Autodesk Inventor part; units mm, degrees
ref_plane "YZ Plane" through (0, 0, 0) normal (1, 0, 0) x (0, 1, 0)
ref_plane "XZ Plane" through (0, 0, 0) normal (0, 1, 0) x (-1, 0, 0)
ref_plane "XY Plane" through (0, 0, 0) normal (0, 0, 1) x (1, 0, 0)
sketch "Sketch6" plane through (0, 0, 0) normal (0, 0, 1) x (1, 0, 0)
  line L0 (40.1, 14.2) -> (56.7, 14.2)
  line L1 (56.7, 14.2) -> (56.7, -14.2)
  line L2 (56.7, -14.2) -> (40.1, -14.2)
  line L3 (40.1, -14.2) -> (40.1, 14.2)
  line L4 (35.6, -18.7) -> (61.2, -18.7)
  line L5 (61.2, -18.7) -> (61.2, 18.7)
  line L6 (61.2, 18.7) -> (35.6, 18.7)
  line L7 (35.6, 18.7) -> (35.6, -18.7)
  line L8 (-40.1, 14.2) -> (-56.7, 14.2)
  line L9 (-56.7, 14.2) -> (-56.7, -14.2)
  line L10 (-56.7, -14.2) -> (-40.1, -14.2)
  line L11 (-40.1, -14.2) -> (-40.1, 14.2)
  line L12 (-35.6, -18.7) -> (-61.2, -18.7)
  line L13 (-61.2, -18.7) -> (-61.2, 18.7)
  line L14 (-61.2, 18.7) -> (-35.6, 18.7)
  line L15 (-35.6, 18.7) -> (-35.6, -18.7)
  point P0 (35.6, 0)
  point P1 (35.6, 0)
  point P2 (-35.6, 0)
  point P3 (-35.6, 0)
extrude "Extrusion4" add sketch "Sketch6" along normal blind 40
sketch "Sketch7" plane through (0, 0, 0) normal (0, 0, -1) x (-1, 0, 0)
  line L0 (-35.6, -18.7) -> (-61.2, -18.7) construction
  line L1 (61.2, 18.7) -> (-61.2, 18.7)
  line L2 (-61.2, 18.7) -> (-61.2, -18.7)
  line L3 (-61.2, -18.7) -> (61.2, -18.7)
  line L4 (61.2, -18.7) -> (61.2, 18.7)
  point P0 (0, 0)
extrude "Extrusion5" add sketch "Sketch7" along normal blind 4.5
sketch "Sketch8" plane through (35.6, 18.7, 40) normal (0, 1, 0) x (1, 0, 0)
  line L0 (-71.2, 40) -> (0, 40) construction
  line L1 (0, 40) -> (0, 0) construction
  line L2 (-25.6, 40) -> (0, 0)
  line L3 (0, 11.1306) -> (-18.4764, 40)
  line L4 (-25.6, 40) -> (-18.4764, 40)
  line L5 (0, 11.1306) -> (0, 0)
  point P0 (-35.6, 40)
extrude "Extrusion6" add sketch "Sketch8" against normal blind 4.5
mirror "Mirror3" about plane through (0, 0, 0) normal (0, 1, 0) of "Extrusion6"
mirror "Mirror4" about plane through (0, 0, 0) normal (1, 0, 0) of "Extrusion6", "Mirror3"
sketch "Sketch9" plane through (0, 0, 0) normal (0, 0, 1) x (1, 0, 0)
  line L0 (12, -18.7) -> (12, -6.7)
  line L1 (-12, -6.7) -> (-12, -18.7)
  line L2 (-35.6, -18.7) -> (-10, -18.7) construction
  line L3 (12, -6.7) -> (-12, -6.7)
  line L4 (12, -18.7) -> (-12, -18.7)
  point P0 (0, 0)
extrude "Extrusion7" cut sketch "Sketch9" along normal mid plane 10
sketch "Sketch10" plane through (0, 0, -4.5) normal (0, 0, -1) x (-1, 0, 0)
  line L0 (12, -6.7) -> (-12, -6.7) construction
  line L1 (10, 18.7) -> (-10, 18.7) construction
  circle A0 centre (0, 12.35) radius 1.8
  circle A1 centre (0, -0.35) radius 1.8
  point P0 (0, 0)
extrude "Extrusion8" cut sketch "Sketch10" against normal blind 10
properties part number "Tablet_joint_Holder"
Model file for the job. Use its own axes, mm. A direction names the side the tool comes from. Coordinates: 2 decimals unless noted, no trailing zeros. Loops run counter-clockwise (first coordinate to the right, second up) from the corner with the lowest first, then second, coordinate; pieces in that order, holes last. Notation, with made-up numbers: (37, -0.5) - (50, -0.5) arc R24 ccw to (50, 31.5) - close; hole circle Ø7 at (70, -30.5). An arc over 180 degrees is marked (long way). Write item = value, one per line. Start each with the question number.
Item 1: Wall check: probe 1 along X at (y, z) = (2.5, 17); probe 2 along Y at (x, z) = (0, -2.5); probe 3 along Y at (x, z) = (31, 23). Give the ranges that are in metal, low to high. Write a range as [from, to].
Item 2: Saw through at B-B, the plane y = -8.5. List the corners of the cut face in (x, z).
Item 3: Drop flat-ended pins along their axis: pin 1 Ø1 at (x, y) = (-42.5, 11.5) entering from +Z; pin 2 Ø12 at (x, y) = (-11.5, -8) entering from -Z. Give the stop position or say it passes through.
Item 4: Saw through at D-D, the plane z = 8. State how many separate pieces and enclosed holes the cut face has, then the cut area to 3 significant figures.
Item 5: Saw through at A-A, the plane z = 32.5. List the corners of the cut face in (x, y), then the cut area to 3 significant figures.
Item 6: Saw through at C-C, the plane x = 0. List the corners of the cut face in (y, z), then the cut area to 3 significant figures.
Item 7: Pull direction Y, two halves, no side cores. Call faces 1 (the face through (-48, 14.2, 20)), 2 (the face through (-61.2, 0, 18)), 3 (the face through (-42, -18.7, 17)): +Y half, -Y half, draft (parallel to the pull), parting line (faces both ways), or undercut.
Item 8: 3-axis set-ups, long thin cutter, end or side, ignore diameter. For faces 4 (the face through (0, 4, 0)), 5 (the face through (-23.63, -16.48, 21.3)), 6 (the face through (49, 0, 0)): which of +Z, -Z, +X, -X, +Y, -Y reach the whole face in a straight line?
Answers:
q1.probe_1 = [-61.2, -56.7], [-40.1, -35.6], [35.6, 40.1], [56.7, 61.2]
q1.probe_2 = [-6.7, -2.15], [1.45, 10.55], [14.15, 18.7]
q1.probe_3 = [-18.7, -14.2], [14.2, 18.7]
q2.outline = (-61.2, -4.5) - (-12, -4.5) - (-12, 0) - (-35.6, 0) - (-35.6, 40) - (-40.1, 40) - (-40.1, 0) - (-56.7, 0) - (-56.7, 40) - (-61.2, 40) - close; (12, -4.5) - (61.2, -4.5) - (61.2, 40) - (56.7, 40) - (56.7, 0) - (40.1, 0) - (40.1, 40) - (35.6, 40) - (35.6, 0) - (12, 0) - close
q3.pin_1 = 0
q3.pin_2 = -4.5
q4.separate_pieces = 6
q4.enclosed_holes = 2
q4.area = 1,100 mm2
q5.outline = (-61.2, -18.7) - (-30.8, -18.7) - (-30.8, -14.2) - (-35.6, -14.2) - (-35.6, 14.2) - (-30.8, 14.2) - (-30.8, 18.7) - (-61.2, 18.7) - close; (30.8, -18.7) - (61.2, -18.7) - (61.2, 18.7) - (30.8, 18.7) - (30.8, 14.2) - (35.6, 14.2) - (35.6, -14.2) - (30.8, -14.2) - close; hole (-56.7, -14.2) - (-40.1, -14.2) - (-40.1, 14.2) - (-56.7, 14.2) - close; hole (40.1, -14.2) - (56.7, -14.2) - (56.7, 14.2) - (40.1, 14.2) - close
q5.area = 1,060 mm2
q6.outline = (-6.7, -4.5) - (-2.15, -4.5) - (-2.15, 0) - (-6.7, 0) - close; (1.45, -4.5) - (10.55, -4.5) - (10.55, 0) - (1.45, 0) - close; (14.15, -4.5) - (18.7, -4.5) - (18.7, 0) - (14.15, 0) - close
q6.area = 81.9 mm2
q7.face_1 = undercut
q7.face_2 = draft
q7.face_3 = -Y half
q8.face_4 = none
q8.face_5 = +Z, +Y, -Y
q8.face_6 = +Z
